Geometry: final body of the model. Coordinates: model frame, mm. Coordinates: 2 decimals unless noted, no trailing zeros. Order: outer loops, then holes, each group sorted by start corner. A loop starts at its lowest first (then second) coordinate and runs counter-clockwise, first axis right, second up. Notation, with made-up numbers: M 8.5,64.5 L 49.5,64.5 A15 cw 49.5,76.5 Z; hole C 43.5,63 d9. An arc over 180 degrees is marked long. Use CSV: the item, a comma, the result in double quotes. Start each with the question number.
1. Material intervals for line 1 (X direction, y = 0.45, z = 11); line 2 (Z direction, x = 10.5, y = 1.8); line 3 (X direction, y = 2.4, z = 1), sorted ascending.
2. Section query D-D on y = 1.4. State how many separate pieces and enclosed holes the cut face has, and give its area (3 significant figures).
3. Pull-direction query (X, two-part tool) for faces 1 (the flat face through (0, 2.54, 3)), 2 (the cylindrical face through (-7.52, 1.29, 11.61)), 3 (the cylindrical face through (-0.15, 1.25, 13.82)), 4 (the cylindrical face through (-15.497, 1.252, -3.441)); classes: pulls with the +X half, pulls with the -X half, needs draft (parallel to the pull), parting line crosses it, or undercut.
4. Section query B-B on x = 0. Return the cut outline in (y, z) (3 decimals), and give its area (3 significant figures).
5. Section query A-A on z = 0. Return the cut outline in (x, y) (3 decimals), and give its area (3 significant figures).
6. Section query C-C on x = -11. Return the cut outline in (y, z), and give its area (3 significant figures).
7. First-contact query: P1, Ø2.5, axis at x = -6.35, z = 11, coming from the -Y side. Flat tip, straight axial feed; report the tip coordinate or a pass-through.
from build123d import *

# Parameters (mm, degrees)
SKETCH1_R                 = 15.875
BOSS_EXTRUDE1_DEPTH       = 2.54
TAP_DRILL_FOR_4_40_TAP1_D = 2.2606
CIRPATTERN1_COUNT         = 6
SKETCH8_R                 = 0.7493
CUT_EXTRUDE1_DEPTH        = 2.54
SKETCH15_R                = 1.3208
CUT_EXTRUDE2_DEPTH        = 2.54
CIRPATTERN2_COUNT         = 6
F_4_40_TAPPED_HOLE3_D     = 2.2606


with BuildPart() as part:
    # Sketch1 → Boss-Extrude1 (new body)
    with BuildSketch(Plane(origin=(0, 0, 0), x_dir=(1, 0, 0), z_dir=(0, 1, 0))):
        with Locations(Location((0, 0, 0), (0, 0, 270))):
            Circle(SKETCH1_R)
    extrude(amount=BOSS_EXTRUDE1_DEPTH)

    # Tap Drill for #4-40 Tap1 (through all)
    with Locations(Plane(origin=(0, 2.54, 0), x_dir=(1, 0, 0), z_dir=(0, 1, 0))):
        with Locations((0, 12.7)):
            tap_drill_for_4_40_tap1 = Hole(TAP_DRILL_FOR_4_40_TAP1_D / 2)

    # CirPattern1: Tap Drill for #4-40 Tap1 ×6 about axis
    cirpattern1_axis = Axis((0, 0, 0), (0, 1, 0))
    for i in range(1, CIRPATTERN1_COUNT):
        add(tap_drill_for_4_40_tap1.rotate(cirpattern1_axis, i * 360 / CIRPATTERN1_COUNT), mode=Mode.SUBTRACT)

    # Sketch8 → Cut-Extrude1 (cut)
    with BuildSketch(Plane(origin=(0, 2.54, 0), x_dir=(1, 0, 0), z_dir=(0, 1, 0))):
        with Locations(Location((0, 0, 0), (0, 0, 270))):
            Circle(SKETCH8_R)
    extrude(amount=-CUT_EXTRUDE1_DEPTH, mode=Mode.SUBTRACT)

    # Sketch15 → Cut-Extrude2 (cut)
    with BuildSketch(Plane(origin=(0, 2.54, 0), x_dir=(1, 0, 0), z_dir=(0, 1, 0))):
        with Locations(Location((12.7, 0, 0), (0, 0, 270))):
            Circle(SKETCH15_R)
    cut_extrude2 = extrude(amount=-CUT_EXTRUDE2_DEPTH, mode=Mode.SUBTRACT)

    # CirPattern2: Cut-Extrude2 ×6 about axis
    cirpattern2_axis = Axis((0, 0, 0), (0, 1, 0))
    for i in range(1, CIRPATTERN2_COUNT):
        add(cut_extrude2.rotate(cirpattern2_axis, i * 360 / CIRPATTERN2_COUNT), mode=Mode.SUBTRACT)

    # #4-40 Tapped Hole3 (through all)
    with Locations(Plane(origin=(0, 2.54, 0), x_dir=(1, 0, 0), z_dir=(0, 1, 0))):
        with Locations((-5.291415217, 3.055)):
            Hole(F_4_40_TAPPED_HOLE3_D / 2)


solid = part.part
Results list:
1,line 1,"x = -11.45 to -7.67, -5.03 to 5.03, 7.67 to 11.45"
1,line 2,"z = -11.91 to -7.36, -5.34 to 5.34, 7.36 to 11.91"
1,line 3,"x = -15.84 to -13.56, -11.84 to 11.84, 13.56 to 15.84"
2,separate pieces,"1"
2,enclosed holes,"14"
2,area,"729 mm²"
3,face 1,"needs draft"
3,face 2,"undercut"
3,face 3,"undercut"
3,face 4,"parting line crosses it"
4,outline,"M 0,-15.875 L 2.54,-15.875 L 2.54,-13.83 L 0,-13.83 Z; M 0,-11.57 L 2.54,-11.57 L 2.54,-0.749 L 0,-0.749 Z; M 0,0.749 L 2.54,0.749 L 2.54,11.57 L 0,11.57 Z; M 0,13.83 L 2.54,13.83 L 2.54,15.875 L 0,15.875 Z"
4,area,"65.4 mm²"
5,outline,"M -15.875,0 L -14.021,0 L -14.021,2.54 L -15.875,2.54 Z; M -11.379,0 L -0.749,0 L -0.749,2.54 L -11.379,2.54 Z; M 0.749,0 L 11.379,0 L 11.379,2.54 L 0.749,2.54 Z; M 14.021,0 L 15.875,0 L 15.875,2.54 L 14.021,2.54 Z"
5,area,"63.4 mm²"
6,outline,"M 0,-11.45 L 2.54,-11.45 L 2.54,-7.48 L 0,-7.48 Z; M 0,-5.22 L 2.54,-5.22 L 2.54,5.22 L 0,5.22 Z; M 0,7.48 L 2.54,7.48 L 2.54,11.45 L 0,11.45 Z"
6,area,"46.7 mm²"
7,P1,"passes through"
